Geometry check sheet. Reference: the model listing, model coordinates, mm. Coordinates: 2 decimals unless noted, no trailing zeros. Write each loop counter-clockwise with the first axis right and the second up, starting at its lowest first coordinate (ties: lowest second). Pieces come first, ordered by that corner, then holes. Notation, with made-up numbers: (-30.5, -6) -> (13.5, -6) arc R21 cw to (13.5, 1) -> close; hole circle Ø8 at (-2.75, 84). An arc over 180 degrees is marked (long way). One line per question, with ' | ' between items.
```python
from build123d import *

# Parameters (mm, degrees)
SKETCH1_R            = 15.24
BOSS_EXTRUDE1_DEPTH  = 1.5875
M3_CLEARANCE_HOLE1_D = 3.4
FILLET1_R            = 5.08
M4_CLEARANCE_HOLE2_D = 4.5
CIRPATTERN1_COUNT    = 3


with BuildPart() as part:
    # Sketch1 → Boss-Extrude1 (new, symmetric)
    with BuildSketch(Plane(origin=(0, 0, 0), x_dir=(1, 0, 0), z_dir=(0, 1, 0))):
        with BuildLine():
            Line((-38.50947489, 32.14883464), (-38.50947489, -32.14883464))
            ThreePointArc((-38.50947489, -32.14883464), (-35.992876625, -34.943383598), (-33.274, -37.541552299))
            Line((-33.274, -37.541552299), (33.274, -37.541552299))
            ThreePointArc((33.274, -37.541552299), (36.035191498, -34.899744966), (38.587271968, -32.055415565))
            Line((38.587271968, -32.055415565), (12.205850338, -14.733372241))
            Line((12.205850338, -14.733372241), (12.205850338, 14.733372241))
            Line((12.205850338, 14.733372241), (38.541369471, 32.110591154))
            ThreePointArc((38.541369471, 32.110591154), (35.567819018, 35.375944868), (32.318597457, 38.367114609))
            Line((32.318597457, 38.367114609), (-32.318597457, 38.367114609))
            ThreePointArc((-32.318597457, 38.367114609), (-35.55025611, 35.393594272), (-38.50947489, 32.14883464))
        make_face()
        with Locations(Location((-15.748, 0, 0), (0, 0, 270))):
            Circle(SKETCH1_R, mode=Mode.SUBTRACT)
    extrude(amount=BOSS_EXTRUDE1_DEPTH, both=True)

    # M3 Clearance Hole1 (through all)
    with Locations(Plane(origin=(0, 1.5875, 0), x_dir=(1, 0, 0), z_dir=(0, 1, 0))):
        with Locations((-33.226947648, 33.226947648), (33.226947648, 33.226947648), (33.226947648, -33.226947648), (-33.226947648, -33.226947648)):
            Hole(M3_CLEARANCE_HOLE1_D / 2)

    # Fillet1
    fillet1_edges = [part.edges().sort_by_distance(p)[0] for p in [
        (12.205850338, 0, -14.733372241),
        (12.205850338, 0, 14.733372241),
    ]]
    fillet(fillet1_edges, radius=FILLET1_R)

    # M4 Clearance Hole2 (through all)
    with Locations(Plane(origin=(0, -1.5875, 0), x_dir=(-1, 0, 0), z_dir=(0, -1, 0))):
        with Locations((-5.752, 0)):
            m4_clearance_hole2 = Hole(M4_CLEARANCE_HOLE2_D / 2)

    # CirPattern1: M4 Clearance Hole2 ×3 about axis
    cirpattern1_axis = Axis((-15.748, 0, 0), (0, 1, 0))
    for i in range(1, CIRPATTERN1_COUNT):
        add(m4_clearance_hole2.rotate(cirpattern1_axis, i * 360 / CIRPATTERN1_COUNT), mode=Mode.SUBTRACT)


solid = part.part
```
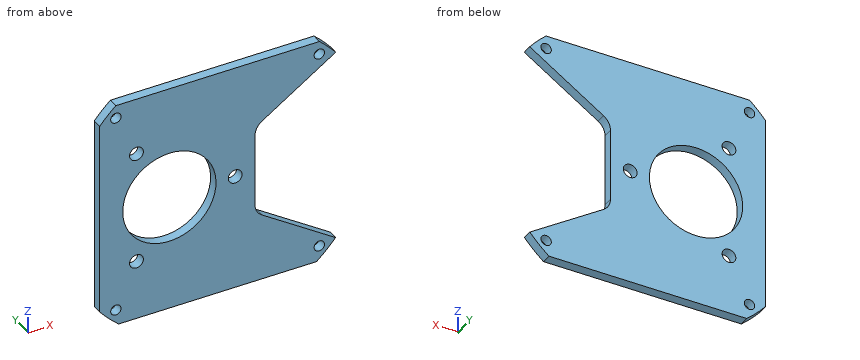
(1) Cross-section at D-D (y = 0.45). Count the separate pieces of the cut face and the enclosed holes in it, plus the area to 3 significant figures.
Answers below:
separate pieces: 1 | enclosed holes: 8 | area: 3,740 mm²
(2) Material ranges on line 1 (Z direction, x = 5.5, y = -1.1); line 2 (Z direction, x = -32, y = -0.9); line 3 (Z direction, x = -27.5, y = 1.05), recorded low to high.
Answers below:
line 1: z = -38.37 to -2.24, 2.24 to 37.54 | line 2: z = -38.37 to -34.4, -32.05 to 32.05, 34.4 to 37.54 | line 3: z = -38.37 to -20.63, -16.6 to -9.7, 9.7 to 16.6, 20.63 to 37.54
(3) Depth check by flat-ended pin: P1, Ø1.5, axis at y = -1, z = -3, coming from the +X side; P2, Ø1, axis at y = 0.5, z = -20.5, coming from the +X side. Enter the tip coordinate at first touch or a pass-through.
Answers below:
P1: stops at x = 12.21 | P2: stops at x = 21.7
(4) Cross-section at A-A (z = 0). Record the cut outline in (x, y).
Answers below:
outline: (-38.51, -1.59) -> (-30.99, -1.59) -> (-30.99, 1.59) -> (-38.51, 1.59) -> close; (-0.51, -1.59) -> (3.5, -1.59) -> (3.5, 1.59) -> (-0.51, 1.59) -> close; (8, -1.59) -> (12.21, -1.59) -> (12.21, 1.59) -> (8, 1.59) -> close
(5) Cross-section at C-C (z = -18). Record the cut outline in (x, y), plus the area to 3 significant figures.
Answers below:
outline: (-38.51, -1.59) -> (-28.66, -1.59) -> (-28.66, 1.59) -> (-38.51, 1.59) -> close; (-24.33, -1.59) -> (17.16, -1.59) -> (17.16, 1.59) -> (-24.33, 1.59) -> close | area: 163 mm²
(6) Cross-section at B-B (x = 16.5). Record the cut outline in (y, z).
Answers below:
outline: (-1.59, -38.37) -> (1.59, -38.37) -> (1.59, -17.57) -> (-1.59, -17.57) -> close; (-1.59, 17.55) -> (1.59, 17.55) -> (1.59, 37.54) -> (-1.59, 37.54) -> close
